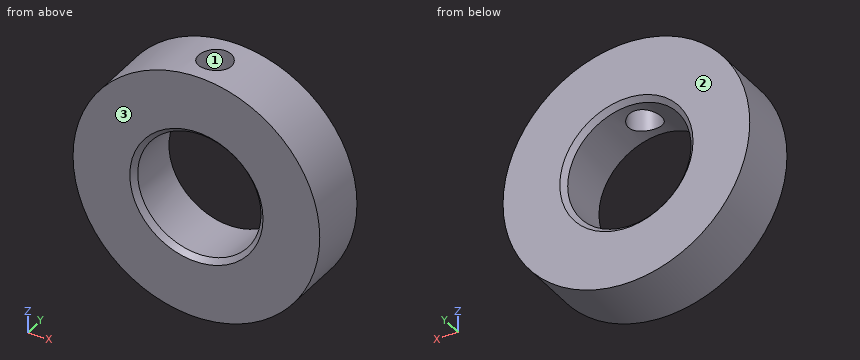
from build123d import *

# Parameters (mm, degrees)
F0_R     = 19.05
F0_R_2   = 9.525
F1_DEPTH = 4.7625
F4_D     = 5.1054
F4_DEPTH = 25.4
F4_START = 0.1718057
F4_TIP   = 1.5338169022
F5_SIZE  = 0.762


with BuildPart() as f1:
    # F0 (on Front) → F1 (new body, symmetric)
    with BuildSketch(Plane.XZ):
        Circle(F0_R)
        Circle(F0_R_2, mode=Mode.SUBTRACT)
    extrude(amount=F1_DEPTH, both=True)

    # F4
    # its depths count from where the whole tool has entered the part; down to there all is cleared
    with Locations(Plane.XY.offset(19.05).offset(-F4_START)):
        with Locations((0, 0)):
            Hole(F4_D / 2, depth=F4_DEPTH)
            with Locations((0, 0, -(F4_DEPTH + F4_TIP / 2))):  # 118° drill point
                Cone(0, F4_D / 2, F4_TIP, mode=Mode.SUBTRACT)

    # F5
    f5_edges = [f1.edges().sort_by_distance(p)[0] for p in [
        (-9.525, -4.7625, 0),
        (-9.525, 4.7625, 0),
    ]]
    chamfer(f5_edges, length=F5_SIZE)


solid = f1.part
Build history of the part. All positions in model axes, mm. Face numbers are marked on the shaded views. Coordinates: 2 decimals unless noted, no trailing zeros. Write each loop counter-clockwise with the first axis right and the second up, starting at its lowest first coordinate (ties: lowest second). Pieces come first, ordered by that corner, then holes.
(1) Cut at A-A on x = 0. State how many separate pieces and enclosed holes the cut face has, and give its area (3 significant figures).
(2) Cut at C-C on y = -3.25. List the corners of the cut face in (x, z) (3 decimals).
(3) Drill centre lines: line 1 (Y direction, x = 0, z = 16.5); line 2 (Z direction, x = 0, y = 1.5) (3 decimals); line 3 (Z direction, x = 8, y = 1.25). Where is each one in solid material? Low to high.
(4) Cut at D-D on y = 0. List the corners of the cut face in (x, z) (3 decimals), and give its area (3 significant figures).
(5) Pin check, flat tips, straight feed: pin 1 Ø2 at (x, z) = (-2.5, -7.5) entering from +Y; pin 2 Ø4 at (y, z) = (-2, -3.5) entering from -X; pin 3 Ø1.5 at (y, z) = (3.5, -9) entering from +X; pin 4 Ø4 at (x, y) = (-8, 0.5) entering from +Z. Stop position of each tip, or through.
(6) Mould opens along Y. For the marked faces 1, 2 and 3 say: pulls with the +Y half, pulls with the -Y half, needs draft (parallel to the pull), parting line crosses it, or undercut.
Working result:
1. separate pieces: 3
1. enclosed holes: 0
1. area: 132 mm2
2. outline: circle Ø38.1 at (0, 0); hole circle Ø19.05 at (0, 0)
3. line 1: y = -4.76 to -2.55, 2.55 to 4.76
3. line 2: z = -19.05 to -9.525
3. line 3: z = -17.29 to -5.17, 5.17 to 17.29
4. outline: (-2.553, 9.177) - (-2.553, 18.878) arc R19.05 ccw (long way) to (2.553, 18.878) - (2.553, 9.177) arc R9.525 cw (long way) to start
4. area: 806 mm2
5. pin 1: passes through
5. pin 2: stops at x = -18.99
5. pin 3: stops at x = 17.17
5. pin 4: stops at z = 18.08
6. face 1: undercut
6. face 2: pulls with the +Y half
6. face 3: pulls with the -Y half
